from build123d import *

# Parameters (mm, degrees)
SKETCH2_W           = 57.5
SKETCH2_H           = 23.5
SKETCH2_R           = 2.5
SKETCH2_W_2         = 40.7
SKETCH2_H_2         = 20.5
BOSS_EXTRUDE1_DEPTH = 2.5
CUT_EXTRUDE1_DEPTH  = 2


with BuildPart() as part:
    # Sketch2 → Boss-Extrude1 (new body)
    with BuildSketch(Plane(origin=(0, 0, 0), x_dir=(1, 0, 0), z_dir=(0, 1, 0))):
        with Locations((-47.929083034, 36.809921321)):
            Rectangle(SKETCH2_W, SKETCH2_H)
        with Locations(Location((-23.429083034, 41.809921321, 0), (0, 0, 270))):
            Circle(SKETCH2_R, mode=Mode.SUBTRACT)
        with Locations(Location((-23.429083034, 31.809921321, 0), (0, 0, 90))):
            Circle(SKETCH2_R, mode=Mode.SUBTRACT)
        with Locations(Location((-72.429083034, 31.809921321, 0), (0, 0, 270))):
            Circle(SKETCH2_R, mode=Mode.SUBTRACT)
        with Locations(Location((-72.429083034, 41.809921321, 0), (0, 0, 90))):
            Circle(SKETCH2_R, mode=Mode.SUBTRACT)
        with Locations((-47.929083034, 36.809921321)):
            Rectangle(SKETCH2_W_2, SKETCH2_H_2, mode=Mode.SUBTRACT)
    extrude(amount=BOSS_EXTRUDE1_DEPTH)

    # Sketch3 → Cut-Extrude1 (cut)
    with BuildSketch(Plane(origin=(0, 2.5, 0), x_dir=(1, 0, 0), z_dir=(0, 1, 0))):
        Polygon((-27.579083034, 36.809921321), (-27.579083034, 36.059921321), (-19.179083034, 36.059921321), (-19.179083034, 37.559921321), (-27.579083034, 37.559921321), align=None)
        Polygon((-76.679083034, 37.559921321), (-68.279083034, 37.559921321), (-68.279083034, 36.809921321), (-68.279083034, 36.059921321), (-76.679083034, 36.059921321), align=None)
    extrude(amount=-CUT_EXTRUDE1_DEPTH, mode=Mode.SUBTRACT)


solid = part.part
The listing builds one solid part. Answer for the finished solid, in the listing's coordinates (mm). A direction names the side the tool comes from. Give positions to 0.01 mm unless a question says otherwise; leave off trailing zeros. Write each loop counter-clockwise with the first axis right and the second up, starting at its lowest first coordinate (ties: lowest second). Pieces come first, ordered by that corner, then holes. Notation, with made-up numbers: (17, 16) -> (73, 16) arc R30 cw to (73, 42) -> close; hole circle Ø11 at (35.5, -6.5). An arc over 180 degrees is marked (long way). One line per question, with ' | ' between items. Start each with the question number.
1. Section B-B (x = -35.5) is taken. Determine the outline of the cut face in (y, z), plus the area to 3 significant figures.
2. For a pull along X with two mould halves and no side action, classify faces 1 (the flat face through (-48, 1, -48.56)), 2 (the cylindrical face through (-23.539, 1.232, -29.312)), 3 (the flat face through (-68.279, 1, -34)), 4 (the flat face through (-76.679, 1, -34)) as pulls with the +X half, pulls with the -X half, needs draft (parallel to the pull), parting line crosses it, or undercut.
3. Given pin 1 Ø2 at (x, z) = (-66, -38) entering from -Y, flat-ended and moving along its own axis, determine where the tip first touches the part or whether it passes through.
4. Section D-D (z = -30.5) is taken. Determine the outline of the cut face in (x, y).
5. Section A-A (y = 1.4) is taken. Determine the outline of the cut face in (x, z).
6. For faces 5 (the flat face through (-27.579, 1, -34)), 6 (the flat face through (-23, 2, -37.56)), 7 (the flat face through (-48, 2.5, -48)), determine the directions among +Z, -Z, +X, -X, +Y, -Y from which every point of the face is accessible in a straight line to the end or side of a thin tool.
7. Find the intervals of material crossed by probe 1 along Z at (x, y) = (-28, 2.15); probe 2 along X at (y, z) = (0.3, -37); probe 3 along Z at (x, y) = (-23, 1.4), in increasing order.
8. Section C-C (z = -37) is taken. Determine the outline of the cut face in (x, y).
Response values:
1) outline: (0, -48.56) -> (2.5, -48.56) -> (2.5, -47.06) -> (0, -47.06) -> close; (0, -26.56) -> (2.5, -26.56) -> (2.5, -25.06) -> (0, -25.06) -> close | area: 7.50 mm2
2) face 1: needs draft | face 2: undercut | face 3: undercut | face 4: pulls with the -X half
3) pin 1: through
4) outline: (-76.68, 0) -> (-74.56, 0) -> (-74.56, 2.5) -> (-76.68, 2.5) -> close; (-70.3, 0) -> (-68.28, 0) -> (-68.28, 2.5) -> (-70.3, 2.5) -> close; (-27.58, 0) -> (-25.56, 0) -> (-25.56, 2.5) -> (-27.58, 2.5) -> close; (-21.3, 0) -> (-19.18, 0) -> (-19.18, 2.5) -> (-21.3, 2.5) -> close
5) outline: (-76.68, -48.56) -> (-19.18, -48.56) -> (-19.18, -37.56) -> (-27.58, -37.56) -> (-27.58, -47.06) -> (-68.28, -47.06) -> (-68.28, -37.56) -> (-76.68, -37.56) -> close; (-76.68, -36.06) -> (-68.28, -36.06) -> (-68.28, -26.56) -> (-27.58, -26.56) -> (-27.58, -36.06) -> (-19.18, -36.06) -> (-19.18, -25.06) -> (-76.68, -25.06) -> close; hole circle Ø5 at (-72.43, -41.81); hole circle Ø5 at (-72.43, -31.81); hole circle Ø5 at (-23.43, -41.81); hole circle Ø5 at (-23.43, -31.81)
6) face 5: +Y, -Y | face 6: +X, -X, +Y | face 7: +Z, -Z, +X, -X, +Y
7) probe 1: -48.56 to -47.06, -26.56 to -25.06 | probe 2: -76.68 to -68.28, -27.58 to -19.18 | probe 3: -48.56 to -44.27, -39.35 to -37.56, -36.06 to -34.27, -29.35 to -25.06
8) outline: (-76.68, 0) -> (-68.28, 0) -> (-68.28, 0.5) -> (-76.68, 0.5) -> close; (-27.58, 0) -> (-19.18, 0) -> (-19.18, 0.5) -> (-27.58, 0.5) -> close
